Could you check a few things on this model? Use its own coordinates, in mm. Face numbers are marked on the shaded views. A direction names the side the tool comes from. Coordinates: 2 decimals unless noted, no trailing zeros. Loops run counter-clockwise (first coordinate to the right, second up) from the corner with the lowest first, then second, coordinate; pieces in that order, holes last. Notation, with made-up numbers: (30, 85) - (57, 85) arc R18 cw to (57, 89) - close; hole circle Ø2 at (37.25, 51). An arc over 180 degrees is marked (long way). One line per question, with ' | ' between items. Start each with the question number.
1. Please list where these lines run through material, in increasing order: L1, parallel to Y at x = 5, z = 7.25; L2, parallel to X at y = 19.5, z = 31.5; L3, parallel to Y at x = 45, z = 7. Write a range as [from, to].
2. We'd pull the mould along X, two halves only. Please class the marked faces 1, 2 and 3: pulls with the +X half, pulls with the -X half, needs draft (parallel to the pull), parting line crosses it, or undercut.
3. I want a section at A-A, the plane z = 12. Write out the boundary of the cut face in (x, y), then the cut area to 3 significant figures.
4. I want a section at B-B, the plane x = 35. Write out the boundary of the cut face in (y, z), then the cut area to 3 significant figures.
5. I want a section at D-D, the plane x = 45. Write out the boundary of the cut face in (y, z), then the cut area to 3 significant figures.
6. I'm going to push flat-ended pins straight in: P1, Ø3.5, axis at x = 34.5, y = 42.5, coming from the +Z side; P2, Ø11, axis at x = 26, y = 24, coming from the +Z side; P3, Ø10, axis at x = 32.5, z = 29, coming from the -Y side; P4, Ø3, axis at x = 8.5, y = 25.5, coming from the -Z side. Where does each tip first touch, or does it pass through?
7. I want a section at C-C, the plane y = 5. Write out the boundary of the cut face in (x, z).
8. Which directions (+Z, -Z, +X, -X, +Y, -Y) give clear straight access to the entire face, cutting with the end or side of a thin tool? Please do the marked faces 4, 5, 6 and 7.
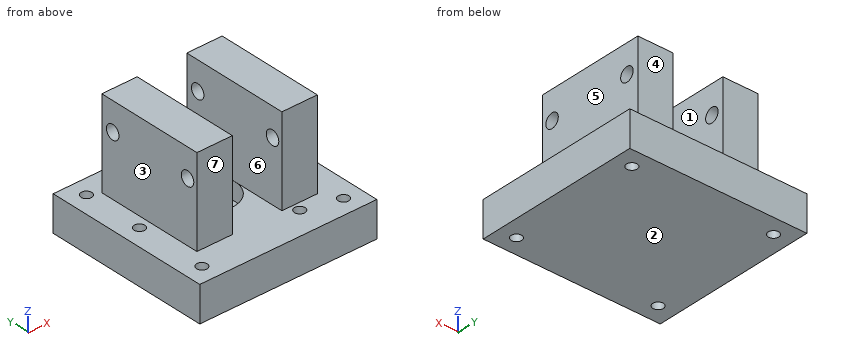
from build123d import *

# Parameters (mm, degrees)
SKETCH_W        = 70
SKETCH_H        = 47
PAD_DEPTH       = 10
SKETCH001_R     = 7
SKETCH001_R_2   = 1.5
POCKET_DEPTH    = 5
SKETCH002_R     = 1.5
SKETCH002_W     = 20
SKETCH002_H     = 70
POCKET001_DEPTH = 10.001
SKETCH003_W     = 10
SKETCH003_H     = 30.5
PAD001_DEPTH    = 25
SKETCH005_R     = 2
POCKET002_DEPTH = 42.001


with BuildPart() as part:
    # Sketch → Pad (new body)
    with BuildSketch(Plane.XY):
        with Locations((35, 23.5)):
            Rectangle(SKETCH_W, SKETCH_H)
    extrude(amount=PAD_DEPTH)

    # Sketch001 → Pocket (cut)
    with BuildSketch(Plane.XY.offset(10)):
        with Locations((25, 25)):
            Circle(SKETCH001_R)
        with Locations((5, 25)):
            Circle(SKETCH001_R_2)
        with Locations((35, 42.320508)):
            Circle(SKETCH001_R_2)
        with Locations((35, 7.679492)):
            Circle(SKETCH001_R_2)
    extrude(amount=-POCKET_DEPTH, mode=Mode.SUBTRACT)

    # Sketch002 → Pocket001 (cut, through all)
    with BuildSketch(Plane.XY.offset(10)):
        with Locations((5, 42)):
            Circle(SKETCH002_R)
        with Locations((5, 5)):
            Circle(SKETCH002_R)
        with Locations((45, 5)):
            Circle(SKETCH002_R)
        with Locations((45, 42)):
            Circle(SKETCH002_R)
        with Locations((60, 15)):
            Rectangle(SKETCH002_W, SKETCH002_H)
    extrude(amount=-POCKET001_DEPTH, mode=Mode.SUBTRACT)

    # Sketch003 → Pad001 (new body)
    with BuildSketch(Plane.XY.offset(10)):
        with Locations((13, 25.25)):
            Rectangle(SKETCH003_W, SKETCH003_H)
        with Locations((37, 25.25)):
            Rectangle(SKETCH003_W, SKETCH003_H)
    extrude(amount=PAD001_DEPTH)

    # Sketch005 → Pocket002 (cut, through all)
    with BuildSketch(Plane.YZ.offset(42)):
        with Locations((13, 27)):
            Circle(SKETCH005_R)
        with Locations((37, 27)):
            Circle(SKETCH005_R)
    extrude(amount=-POCKET002_DEPTH, mode=Mode.SUBTRACT)


solid = part.part
Results are:
1) L1: y = [0, 3.5], [6.5, 23.5], [26.5, 40.5], [43.5, 47] | L2: x = [8, 18], [32, 42] | L3: y = [0, 3.5], [6.5, 40.5], [43.5, 47]
2) face 1: undercut | face 2: needs draft | face 3: pulls with the -X half
3) outline: (8, 10) - (18, 10) - (18, 40.5) - (8, 40.5) - close; (32, 10) - (42, 10) - (42, 40.5) - (32, 40.5) - close | area: 610 mm2
4) outline: (0, 0) - (47, 0) - (47, 10) - (43.82, 10) - (43.82, 5) - (40.82, 5) - (40.82, 10) - (40.5, 10) - (40.5, 35) - (10, 35) - (10, 10) - (9.18, 10) - (9.18, 5) - (6.18, 5) - (6.18, 10) - (0, 10) - close; hole circle Ø4 at (13, 27); hole circle Ø4 at (37, 27) | area: 1,180 mm2
5) outline: (0, 0) - (3.5, 0) - (3.5, 10) - (0, 10) - close; (6.5, 0) - (40.5, 0) - (40.5, 10) - (6.5, 10) - close; (43.5, 0) - (47, 0) - (47, 10) - (43.5, 10) - close | area: 410 mm2
6) P1: stops at z = 10 | P2: stops at z = 5 | P3: stops at y = 10 | P4: stops at z = 0
7) outline: (0, 0) - (3.5, 0) - (3.5, 10) - (0, 10) - close; (6.5, 0) - (43.5, 0) - (43.5, 10) - (6.5, 10) - close; (46.5, 0) - (50, 0) - (50, 10) - (46.5, 10) - close
8) face 4: +Z, +X, -X, +Y | face 5: +Z, +X, +Y, -Y | face 6: +Z, +Y, -Y | face 7: +Z, +X, -X, -Y
